Could you check a few things on this model? Use its own coordinates, in mm. A direction names the side the tool comes from. Give positions to 0.01 mm unless a question says otherwise; leave off trailing zeros. Order: outer loops, then holes, each group sorted by start corner. A loop starts at its lowest first (then second) coordinate and runs counter-clockwise, first axis right, second up. Notation, with made-up numbers: (-32, 58.5) -> (-15, 58.5) arc R24 ccw to (-15, 85.5) -> close; hole circle Ø11 at (-26.75, 27). An arc over 180 degrees is marked (long way). Answer as CSV lines item,"result". Start each with the question number.
(1) On a 3-axis mill with a long thin cutter (end or side, diameter ignored), from which of +Z, -Z, +X, -X, +Y, -Y can I reach the whole of each face in a straight line? I mean faces 1 (the face through (3.35, -98.93, 3.01)), 2 (the face through (11.3, -92, 15)). Say none if no direction works.
(2) I want a section at A-A (x = 11). Please give me the cut outline in (y, z), plus the area to 3 significant figures.
(3) I want a section at D-D (y = -93.75). Please give me the cut outline in (x, z), plus the area to 3 significant figures.
(4) I need wall thicknesses on L1, parallel to Y at x = 9.75, z = 12.25; L2, parallel to Z at x = 5.75, y = -98; L3, parallel to X at y = -90.75, z = 9.75. Which ranges of each line are inside material? Lowest first, please.
(5) We'd pull the mould along X, two halves only. Please class faces 3 (the face through (1.4, -98.7, 2)), 4 (the face through (4.137, -90.56, 1.972)), 5 (the face through (6, -97, 2)), 6 (the face through (6.3, -93.7, 4)): released by +X, released by -X, zero draft, split by the parting line, or undercut.
(6) I want a section at C-C (x = 6.25). Please give me the cut outline in (y, z), plus the area to 3 significant figures.
(7) I want a section at B-B (y = -91.75). Please give me the cut outline in (x, z).
(8) Will these pins go through, and if not, where does the flat tip stop? pin 1 Ø1 at (y, z) = (-90.5, 2.5) entering from -X; pin 2 Ø3 at (x, y) = (9.66, -90.34) entering from +Z; pin 3 Ø5 at (x, z) = (6, 7) entering from -Y; pin 4 Ø2 at (y, z) = (-93.5, 13.5) entering from -X.
```python
from build123d import *

# Parameters (mm, degrees)
SKETCH2_R           = 2
BOSS_EXTRUDE1_DEPTH = 4
SKETCH3_R           = 2
CUT_EXTRUDE1_DEPTH  = 4
SKETCH4_R           = 3
CUT_EXTRUDE2_DEPTH  = 2
SKETCH5_R           = 3.75
SKETCH5_R_2         = 2
BOSS_EXTRUDE2_DEPTH = 11


with BuildPart() as part:
    # Sketch2 → Boss-Extrude1 (new body)
    with BuildSketch(Plane.XY):
        with BuildLine():
            Line((1.348357032, -93.348542262), (7.005211484, -87.691688216))
            ThreePointArc((7.005211484, -87.691688216), (12.308512224, -87.691688287), (12.308512391, -92.994989027))
            Line((12.308512391, -92.994989027), (6.651658446, -98.651843581))
            ThreePointArc((6.651658446, -98.651843581), (1.348356961, -98.651843747), (1.348357032, -93.348542262))
        make_face()
        with Locations((9.656861819, -90.34333874)):
            Circle(SKETCH2_R, mode=Mode.SUBTRACT)
    extrude(amount=BOSS_EXTRUDE1_DEPTH)

    # Sketch3 → Cut-Extrude1 (cut)
    with BuildSketch(Plane.XY.offset(4)):
        with Locations((4.00000762, -96.00019304)):
            Circle(SKETCH3_R)
    extrude(amount=-CUT_EXTRUDE1_DEPTH, mode=Mode.SUBTRACT)

    # Sketch4 → Cut-Extrude2 (cut)
    with BuildSketch(Plane.XY.offset(4)):
        with Locations((4.00000762, -96.00019304)):
            Circle(SKETCH4_R)
    extrude(amount=-CUT_EXTRUDE2_DEPTH, mode=Mode.SUBTRACT)

    # Sketch5 → Boss-Extrude2 (add)
    with BuildSketch(Plane.XY.offset(4)):
        with Locations((9.656861819, -90.34333874)):
            Circle(SKETCH5_R)
        with Locations((9.656861819, -90.34333874)):
            Circle(SKETCH5_R_2, mode=Mode.SUBTRACT)
    extrude(amount=BOSS_EXTRUDE2_DEPTH)


solid = part.part
```
Final values:
1,face 1,"+Z"
1,face 2,"+Z, +X, -X, +Y, -Y"
2,outline,"(-94.3, 0) -> (-91.83, 0) -> (-91.83, 15) -> (-93.84, 15) -> (-93.84, 4) -> (-94.3, 4) -> close; (-88.86, 0) -> (-86.84, 0) -> (-86.84, 15) -> (-88.86, 15) -> close"
2,area,"62.4 mm²"
3,outline,"(1, 0) -> (11.55, 0) -> (11.55, 4) -> (11.22, 4) -> (11.22, 15) -> (8.09, 15) -> (8.09, 4) -> (5.98, 4) -> (5.98, 2) -> (2.02, 2) -> (2.02, 4) -> (1, 4) -> close"
3,area,"68.8 mm²"
4,L1,"-94.09 to -92.34, -88.35 to -86.59"
4,L2,"0 to 2"
4,L3,"5.93 to 7.7, 11.62 to 13.38"
5,face 3,"split by the parting line"
5,face 4,"released by -X"
5,face 5,"undercut"
5,face 6,"zero draft"
6,outline,"(-99, 0) -> (-88.45, 0) -> (-88.45, 4) -> (-88.78, 4) -> (-88.78, 15) -> (-91.91, 15) -> (-91.91, 4) -> (-94.02, 4) -> (-94.02, 2) -> (-97.98, 2) -> (-97.98, 4) -> (-99, 4) -> close"
6,area,"68.8 mm²"
7,outline,"(2.95, 0) -> (8.24, 0) -> (8.24, 15) -> (6.18, 15) -> (6.18, 4) -> (2.95, 4) -> close; (11.08, 0) -> (13.13, 0) -> (13.13, 15) -> (11.08, 15) -> close"
8,pin 1,"x = 3.7"
8,pin 2,"through"
8,pin 3,"y = -93.91"
8,pin 4,"x = 6.59"
